Geometry check sheet. Reference: the model listing, model coordinates, mm. A direction names the side the tool comes from. Coordinates: 2 decimals unless noted, no trailing zeros. Write each loop counter-clockwise with the first axis right and the second up, starting at its lowest first coordinate (ties: lowest second). Pieces come first, ordered by that corner, then holes. Notation, with made-up numbers: (56.25, 5.5) -> (94.25, 5.5) arc R15 ccw to (94.25, 29.5) -> close; hole circle Ø8 at (70, -9.5). An arc over 180 degrees is marked (long way). Use a Markdown table: item, result.
```python
from build123d import *

# Parameters (mm, degrees)
F0_W          = 66
F0_H          = 25.4
F1_DEPTH      = 5.2
F2_W          = 20
F2_H          = 20
F3_DEPTH      = 2
F4_R          = 7
F5_DEPTH      = 16.04009
F6_R          = 1
F7_DEPTH      = 25
F7_DEPTH_BACK = 25


with BuildPart() as f1:
    # F0 (on Top) → F1 (new body)
    with BuildSketch(Plane.XY):
        Rectangle(F0_W, F0_H)
    extrude(amount=F1_DEPTH)

    # F2 (on face) → F3 (join)
    with BuildSketch(Plane.XY.offset(5.2)):
        Rectangle(F2_W, F2_H)
    extrude(amount=F3_DEPTH)

    # F4 (on face) → F5 (cut)
    with BuildSketch(Plane.XY.offset(7.2)):
        Circle(F4_R)
    extrude(amount=-F5_DEPTH, mode=Mode.SUBTRACT)

    # F6 (on Front) → F7 (cut, two sides)
    with BuildSketch(Plane.XZ) as f7_sk:
        with Locations((31.872865, 0)):
            Circle(F6_R)
    extrude(amount=F7_DEPTH, mode=Mode.SUBTRACT)
    extrude(f7_sk.sketch, amount=-F7_DEPTH_BACK, mode=Mode.SUBTRACT)


solid = f1.part
```
Item 1: Section check C-C on x = -9. Record the boundary of the cut face in (y, z), then the cut area to 3 significant figures.
Answer block:
| item | result |
|---|---|
| outline | (-12.7, 0) -> (12.7, 0) -> (12.7, 5.2) -> (10, 5.2) -> (10, 7.2) -> (-10, 7.2) -> (-10, 5.2) -> (-12.7, 5.2) -> close |
| area | 172 mm^2 |
Item 2: Thickness scan on L1, parallel to Y at x = 0, z = 4; L2, parallel to Z at x = -8, y = 10.5; L3, parallel to X at y = -3.25, z = 3. Record the ranges inside material, lowest first. Write a range as [from, to].
Answer block:
| item | result |
|---|---|
| L1 | y = [-12.7, -7], [7, 12.7] |
| L2 | z = [0, 5.2] |
| L3 | x = [-33, -6.2], [6.2, 33] |
Item 3: Depth check by flat-ended pin: P1, Ø0.6, axis at y = -2, z = 6.5, coming from the +X side; P2, Ø2, axis at x = -2, z = 6.5, coming from the -Y side; P3, Ø1, axis at x = 21.5, y = 7.5, coming from the +Z side. Enter the tip coordinate at first touch or a pass-through.
Answer block:
| item | result |
|---|---|
| P1 | stops at x = 10 |
| P2 | stops at y = -10 |
| P3 | stops at z = 5.2 |
Item 4: Section check B-B on y = -4.75. Record the boundary of the cut face in (x, z), then the cut area to 3 significant figures.
Answer block:
| item | result |
|---|---|
| outline | (-33, 0) -> (-5.14, 0) -> (-5.14, 7.2) -> (-10, 7.2) -> (-10, 5.2) -> (-33, 5.2) -> close; (5.14, 0) -> (30.87, 0) arc R1 cw to (32.87, 0) -> (33, 0) -> (33, 5.2) -> (10, 5.2) -> (10, 7.2) -> (5.14, 7.2) -> close |
| area | 308 mm^2 |
Item 5: Tool access check on faces 1 (the flat face through (10, 0, 6)), 2 (the flat face through (0, 10, 6)), 3 (the flat face through (0, -10, 6)). Record the directions out of +Z, -Z, +X, -X, +Y, -Y that give a thin tool (end or side, any length) a straight path to the whole face; none if there is none.
Answer block:
| item | result |
|---|---|
| face 1 | +Z, +X, +Y, -Y |
| face 2 | +Z, +X, -X, +Y |
| face 3 | +Z, +X, -X, -Y |
Item 6: Section check A-A on x = 0. Record the boundary of the cut face in (y, z).
Answer block:
| item | result |
|---|---|
| outline | (-12.7, 0) -> (-7, 0) -> (-7, 7.2) -> (-10, 7.2) -> (-10, 5.2) -> (-12.7, 5.2) -> close; (7, 0) -> (12.7, 0) -> (12.7, 5.2) -> (10, 5.2) -> (10, 7.2) -> (7, 7.2) -> close |
Item 7: Section check D-D on z = 4.25. Record the boundary of the cut face in (x, y).
Answer block:
| item | result |
|---|---|
| outline | (-33, -12.7) -> (33, -12.7) -> (33, 12.7) -> (-33, 12.7) -> close; hole circle Ø14 at (0, 0) |
